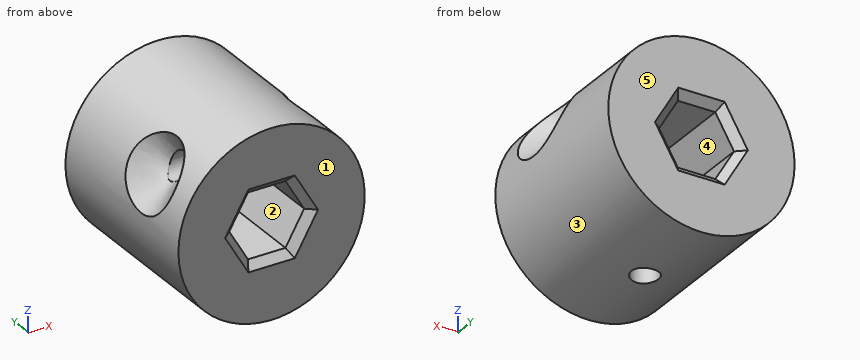
Autodesk Inventor part; units mm, degrees
ref_plane "Work Plane2" through (0, 0, -19.05) normal (0, 0, 1) x (1, 0, 0)
ref_plane "YZ Plane" through (0, 0, 0) normal (1, 0, 0) x (0, 1, 0)
ref_plane "XZ Plane" through (0, 0, 0) normal (0, 1, 0) x (-1, 0, 0)
sketch "Sketch9" plane through (0, 0, 0) normal (0, 1, 0) x (-1, 0, 0)
  circle A0 centre (0, 0) radius 19.05
  dimension "d53" = 38.1
extrude "Extrusion6" add sketch "Sketch9" along normal mid plane 36.8554
sketch "Sketch10" plane through (0, 18.4277, 0) normal (0, 1, 0) x (1, 0, 0)
  circle A0 centre (0, 0) radius 13.589
  dimension "idWasher" = 27.178
extrude "Extrusion7" add sketch "Sketch10" along normal blind 2.3707
sketch "Sketch11" plane through (0, 20.7984, 0) normal (0, 1, 0) x (1, 0, 0)
  line L0 (7.6623, 0) -> (3.8312, -6.6358)
  line L1 (3.8312, -6.6358) -> (-3.8312, -6.6358)
  line L2 (-3.8312, -6.6358) -> (-7.6623, 0)
  line L3 (-7.6623, 0) -> (-3.8312, 6.6357)
  line L4 (-3.8312, 6.6357) -> (3.8312, 6.6357)
  line L5 (3.8312, 6.6357) -> (7.6623, 0)
  point P0 (0, 0)
  point P1 (0, 0)
  dimension "d59" = 13.2715
extrude "Extrusion8" cut sketch "Sketch11" against normal through all
sketch "Sketch12" plane through (0, 0, 0) normal (1, 0, 0) x (0, 1, 0)
  circle A0 centre (-6.1426, 9.1758) radius 2.54
  line L0 (20.7984, 0) -> (-18.4277, 0)
  line L1 (-18.4277, 19.05) -> (-18.4277, -19.05)
  point P0 (0, 0)
  dimension "d62" = 5.08
  dimension "d63" = 9.1758
  dimension "oneThirdSpoolHeight" = 12.2851
extrude "Extrusion9" cut sketch "Sketch12" along normal through all both and the other way through all
chamfer "Chamfer5" distance 4.7625 angle 45 2 edges at (16.6229, -8.6793, 9.3048) (-16.6229, -8.6793, 9.3048)
ref_plane "Work Plane2" through (0, 0, -19.05) normal (0, 0, 1) x (1, 0, 0)
sketch "Sketch13" plane through (0, 0, -19.05) normal (0, 0, 1) x (1, 0, 0)
  point P0 (0, 0)
  point P1 (0, 0)
hole "Hole2" at (0, 0, -19.05) direction (0, 0, 1) diameter 4.699 depth 12.4143 counterbore diameter 5.5372 counterbore depth 5.5626
chamfer "Chamfer6" distance 1.5875 angle 45 12 edges at (-5.7467, 20.7984, -3.3179) (0, 20.7984, -6.6357) (5.7467, 20.7984, -3.3179) (5.7467, 20.7984, 3.3179) (0, 20.7984, 6.6358) (-5.7467, 20.7984, 3.3179) (0, -18.4277, 6.6358) (5.7467, -18.4277, 3.3179) (5.7467, -18.4277, -3.3179) (0, -18.4277, -6.6357) (-5.7467, -18.4277, -3.3179) (-5.7467, -18.4277, 3.3179)
sketch "Sketch14" plane through (0, 20.7984, 0) normal (0, 1, 0) x (1, 0, 0)
  circle A0 centre (0, 0) radius 19.05
extrude "Extrusion10" cut sketch "Sketch14" against normal blind 2.413
chamfer "Chamfer7" distance 1.5875 angle 45 6 edges at (-5.7467, 18.3854, -3.3179) (0, 18.3854, -6.6357) (5.7467, 18.3854, -3.3179) (5.7467, 18.3854, 3.3179) (0, 18.3854, 6.6358) (-5.7467, 18.3854, 3.3179)
equation "\"d53\" = spoolInteriorDiameter"
equation "\"d59\" = hexDiameter"
equation "\"d62\" = holeForString"
equation "\"d63\" = stringHoleCenterFromHexShaft"
equation "\"oneThirdSpoolHeight\" = 0.333333 * singleSpoolHeight"
equation "\"d67\" = stringHoleChamfer"
equation "\"d77\" = hexHoleChamfer"
equation "\"d82\" = hexHoleChamfer"
equation "\"holeForString\" = stringDiameter + clearanceForString"
equation "\"stringDiameter\" = 3.048"
equation "\"clearanceForString\" = 2.032"
equation "\"spoolHeightWithoutSpacer\" = 69.85"
equation "\"hexShaftDiameter\" = 12.7"
equation "\"clearanceForHexShaft\" = 0.5715"
equation "\"hexDiameter\" = hexShaftDiameter + clearanceForHexShaft"
equation "\"supportChannels\" = 3.81"
equation "\"spoolInteriorDiameter\" = 38.1"
equation "\"spoolInteriroRadius\" = 0.5 * spoolInteriorDiameter"
equation "\"spoolExteriorDiameter\" = 88.9"
equation "\"spoolExteriorRadius\" = 0.5 * spoolExteriorDiameter"
equation "\"spoolFiletRadius\" = 0.5 * supportChannels"
equation "\"holeCenter\" = 0.25 * spoolHeightWithoutSpacer - 0.75 * supportChannels"
equation "\"hexHoleChamfer\" = 1.5875"
equation "\"stringHoleCenterFromHexShaft\" = 0.5 * hexDiameter + 0.5 * holeForString"
equation "\"textCircleDiameter\" = 0.75 * spoolExteriorDiameter"
equation "\"textHeight\" = 6.096"
equation "\"textDepth\" = 1.27"
equation "\"stringHoleChamfer\" = 4.7625"
equation "\"spoolTotalHeight\" = 76.2"
equation "\"spaceHeight\" = spoolTotalHeight - spoolHeightWithoutSpacer"
equation "\"spacerDiameter\" = 24.13"
properties part number "spoolV05" material "PC/ABS Plastic"
Check sheet for the modelled part. Datum: model origin and axes. Units: mm. Face numbers are marked on the shaded views. A direction names the side the tool comes from. Give positions to 0.01 mm unless a question says otherwise; leave off trailing zeros. Loops run counter-clockwise (first coordinate to the right, second up) from the corner with the lowest first, then second, coordinate; pieces in that order, holes last. Notation, with made-up numbers: M 71,43 L 95,43 A14 cw 95,47 Z; hole C -24,81 d4. An arc over 180 degrees is marked long. Use a Markdown table: item, result. Add a question column.
Q1. Sectioned sample at D-D, the plane y = -7. Give the number of separate pieces and of enclosed holes in the cut face, then the cut area to 3 significant figures.
Q2. Tool access check on the marked faces 1 and 2. Record the directions out of +Z, -Z, +X, -X, +Y, -Y that give a thin tool (end or side, any length) a straight path to the whole face; none if there is none.
Q3. Mould release check, pull along X, two halves, no side actions. Record for the marked faces 3, 4 and 5: pulls with the +X half, pulls with the -X half, needs draft (parallel to the pull), parting line crosses it, or undercut.
Q4. Sectioned sample at C-C, the plane y = 10. Record the cut outline in (x, z), then the cut area to 3 significant figures.
Q5. Sectioned sample at B-B, the plane z = -4. Record the cut outline in (x, y).
Q6. Go/stop test with flat-tipped pins: pin 1 (2 mm diameter, centred on x = -3, y = 11, fed in from -Z); pin 2 (1.5 mm diameter, centred on y = -11.5, z = 10, fed in from +X); pin 3 (5 mm diameter, centred on x = -14, y = -1, fed in from +Z); pin 4 (3 mm diameter, centred on y = -6.14, z = 9.18, fed in from -X). Record where each tip stops, or that it passes through.
Q7. Sectioned sample at A-A, the plane x = 0. Record the cut outline in (y, z), then the cut area to 3 significant figures.
Q8. Scan lines: line 1 along Y through (x, z) = (0, -15.75); line 2 along Y through (x, z) = (0, -8.25); line 3 along Z through (x, y) = (0, -1.5). Record each from-to range of solid material in increasing order. Write a range as [from, to].
Verdict:
| question | item | result |
|---|---|---|
| 1 | separate pieces | 2 |
| 1 | enclosed holes | 1 |
| 1 | area | 787 mm^2 |
| 2 | face 1 | +Z, -Z, +X, -X, -Y |
| 2 | face 2 | +Y, -Y |
| 3 | face 3 | parting line crosses it |
| 3 | face 4 | undercut |
| 3 | face 5 | needs draft |
| 4 | outline | C 0,0 d38.1; hole M -7.66,0 L -3.83,-6.64 L 3.83,-6.64 L 7.66,0 L 3.83,6.64 L -3.83,6.64 Z |
| 4 | area | 988 mm^2 |
| 5 | outline | M -18.63,-18.43 L -7.19,-18.43 L -5.35,-16.84 L -5.35,16.8 L -7.19,18.39 L -18.63,18.39 Z; M 5.35,-16.84 L 7.19,-18.43 L 18.63,-18.43 L 18.63,18.39 L 7.19,18.39 L 5.35,16.8 Z |
| 6 | pin 1 | z = -18.94 |
| 6 | pin 2 | x = 15.29 |
| 6 | pin 3 | z = 15.19 |
| 6 | pin 4 | through |
| 7 | outline | M -18.43,-19.05 L -2.77,-19.05 L -2.77,-13.49 L -2.35,-13.49 L -2.35,-6.64 L -16.84,-6.64 L -18.43,-8.22 Z; M -18.43,8.22 L -16.84,6.64 L 16.8,6.64 L 18.39,8.22 L 18.39,19.05 L -18.43,19.05 Z; M 2.35,-13.49 L 2.77,-13.49 L 2.77,-19.05 L 18.39,-19.05 L 18.39,-8.22 L 16.8,-6.64 L 2.35,-6.64 Z; hole C -6.14,9.18 d5.08 |
| 7 | area | 826 mm^2 |
| 8 | line 1 | [-18.43, -2.77], [2.77, 18.39] |
| 8 | line 2 | [-18.43, -2.35], [2.35, 18.39] |
| 8 | line 3 | [6.64, 19.05] |
